Could you check a few things on this drawing? It's one solid part, dimensions in mm from its lowest x, y, z. Give positions to 0.01 mm unless a question says otherwise; leave off trailing zeros. Order: outer loops, then holes, each group sorted by start corner. A loop starts at its lowest first (then second) coordinate and runs counter-clockwise, first axis right, second up.
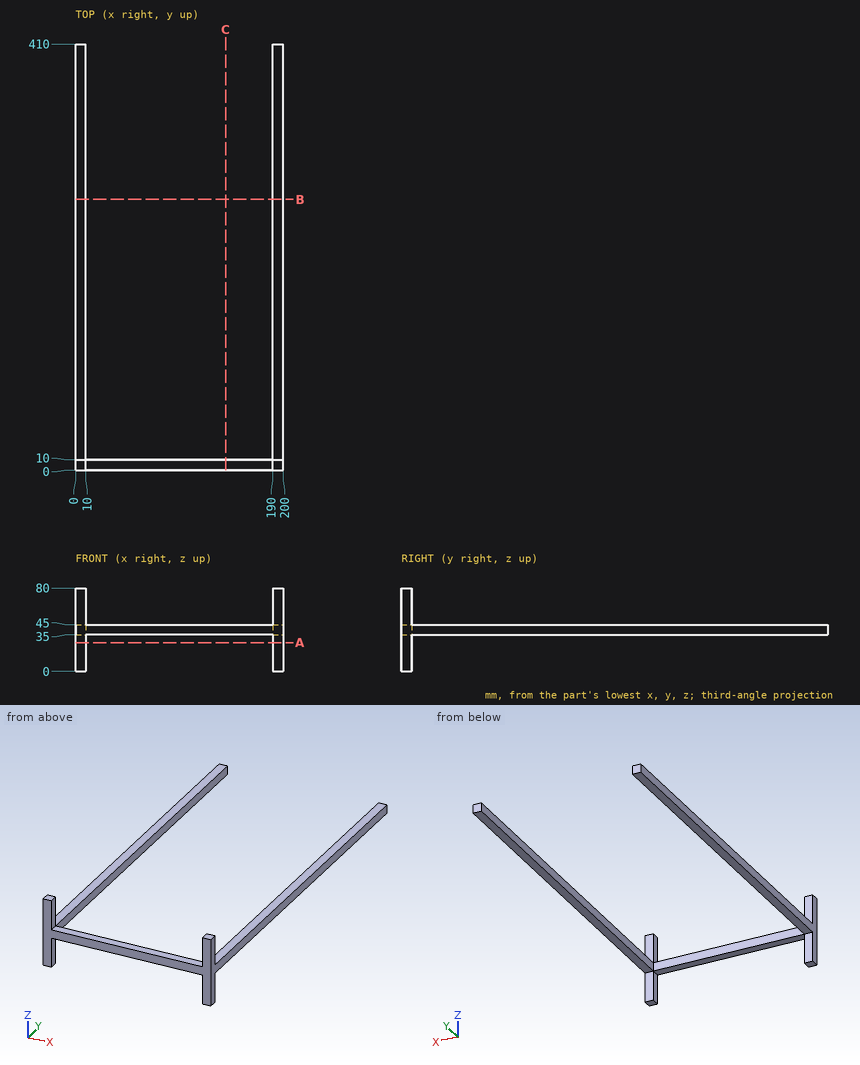
Q1. If we section it at B-B on y = 260.5: List the corners of the cut face in (x, z) for me.
Filled sheet:
outline: (0, 35) - (10, 35) - (10, 45) - (0, 45) - close; (190, 35) - (200, 35) - (200, 45) - (190, 45) - close
Q2. If we section it at C-C on x = 144.5: List the corners of the cut face in (y, z) for me, plus the area to 3 significant figures.
Filled sheet:
outline: (0, 35) - (10, 35) - (10, 45) - (0, 45) - close
area: 100 mm2
Q3. I'm going to push flat-ended pins straight in: P1, Ø3, axis at x = 194, z = 70, coming from the +Y side; P2, Ø8, axis at x = 5.5, y = 186.5, coming from the -Z side; P3, Ø11, axis at x = 193.5, y = 115, coming from the +Z side; P4, Ø10, axis at y = 361.5, z = 38.5, coming from the -X side. Where does each tip first touch, or does it pass through?
Filled sheet:
P1: stops at y = 10
P2: stops at z = 35
P3: stops at z = 45
P4: stops at x = 0
Q4. If we section it at A-A on z = 27.5: List the corners of the cut face in (x, y) for me, plus the area to 3 significant figures.
Filled sheet:
outline: (0, 0) - (10, 0) - (10, 10) - (0, 10) - close; (190, 0) - (200, 0) - (200, 10) - (190, 10) - close
area: 200 mm2
Q5. I need wall thicknesses on L1, parallel to X at y = 391.5, z = 44. Which ranges of the line are inside material? Lowest first, please.
Filled sheet:
L1: x = 0 to 10, 190 to 200
